Input: dimensioned drawing with shaded views. Units: mm. Origin: part minimum x, y, z. Give positions to 0.01 mm unless a question says otherwise; leave off trailing zeros. Order: outer loops, then holes, each group sorted by start corner. A loop starts at its lowest first (then second) coordinate and runs counter-clockwise, first axis right, second up. Notation, with made-up numbers: (23.5, 71.5) - (70.5, 71.5) arc R19 ccw to (70.5, 91.5) - close; hole circle Ø10 at (-1.75, -23.5). An arc over 180 degrees is marked (long way). Use a Markdown table: item, result.
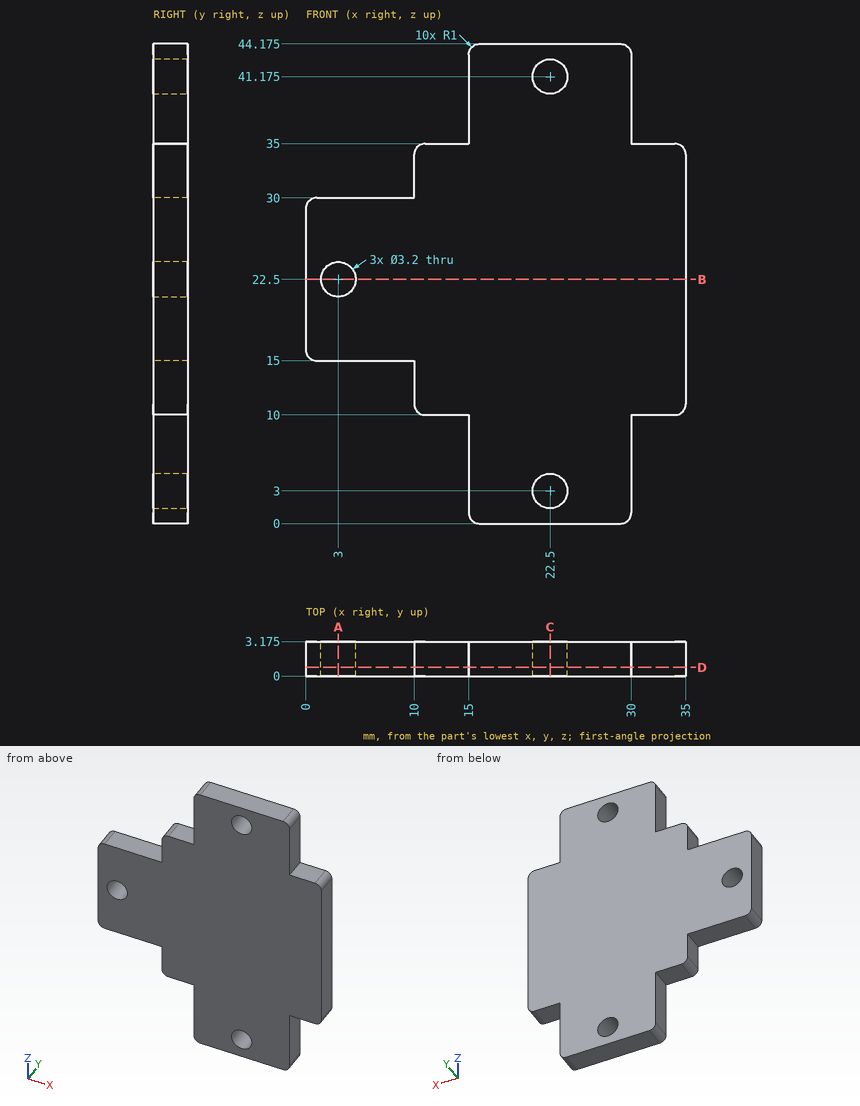
1. Section query C-C (x = 22.5). Return loops of the section in (y, z) (3 decimals), then the cut area to 3 significant figures.
Response:
| item | result |
|---|---|
| outline | (0, 0) - (3.175, 0) - (3.175, 1.4) - (0, 1.4) - close; (0, 4.6) - (3.175, 4.6) - (3.175, 39.575) - (0, 39.575) - close; (0, 42.775) - (3.175, 42.775) - (3.175, 44.175) - (0, 44.175) - close |
| area | 120 mm^2 |
2. Section query B-B (z = 22.5). Return loops of the section in (x, y) (3 decimals), then the cut area to 3 significant figures.
Response:
| item | result |
|---|---|
| outline | (0, 0) - (1.4, 0) - (1.4, 3.175) - (0, 3.175) - close; (4.6, 0) - (35, 0) - (35, 3.175) - (4.6, 3.175) - close |
| area | 101 mm^2 |
3. Section query A-A (x = 3). Return loops of the section in (y, z) (3 decimals).
Response:
| item | result |
|---|---|
| outline | (0, 15) - (3.175, 15) - (3.175, 20.9) - (0, 20.9) - close; (0, 24.1) - (3.175, 24.1) - (3.175, 30) - (0, 30) - close |
4. Pin query (flat end, axial travel): pin 1 (4 mm diameter, centred on x = 3, z = 22.5, fed in from -Y); pin 2 (1 mm diameter, centred on y = 1, z = 5.5, fed in from -X); pin 3 (1.9 mm diameter, centred on x = 22.5, z = 3, fed in from -Y); pin 4 (1 mm diameter, centred on y = 2, z = 39, fed in from +X). Return the tip coordinate at first contact, or that it passes through.
Response:
| item | result |
|---|---|
| pin 1 | stops at y = 0 |
| pin 2 | stops at x = 15 |
| pin 3 | passes through |
| pin 4 | stops at x = 30 |
5. Material intervals for line 1 along X through (y, z) = (0.7, 3); line 2 along X through (y, z) = (1.85, 30.5); line 3 along X through (y, z) = (2.9, 38.5), sorted ascending.
Response:
| item | result |
|---|---|
| line 1 | x = 15 to 20.9, 24.1 to 30 |
| line 2 | x = 10 to 35 |
| line 3 | x = 15 to 30 |
6. Section query D-D (y = 0.8). State how many separate pieces and enclosed holes the cut face has, then the cut area to 3 significant figures.
Response:
| item | result |
|---|---|
| separate pieces | 1 |
| enclosed holes | 3 |
| area | 1,040 mm^2 |
